from build123d import *

# Parameters (mm, degrees)
SKETCH1_W      = 11.90625
SKETCH1_H      = 34.925
EXTRUDE1_DEPTH = 1.984375
SKETCH4_W      = 11.90625
SKETCH4_H      = 11.303912273
EXTRUDE3_DEPTH = 0.79375
SKETCH2_R      = 2.1
EXTRUDE2_DEPTH = 1.984375
CHAMFER1_SIZE  = 0.508


with BuildPart() as part:
    # Sketch1 → Extrude1 (new body)
    with BuildSketch(Plane(origin=(0, 0, 0), x_dir=(1, 0, 0), z_dir=(0, 1, 0))):
        Rectangle(SKETCH1_W, SKETCH1_H)
    extrude(amount=EXTRUDE1_DEPTH)

    # Sketch4 → Extrude3 (cut)
    with BuildSketch(Plane.XZ):
        with Locations((0, 11.810543864)):
            Rectangle(SKETCH4_W, SKETCH4_H)
    extrude3 = extrude(amount=-EXTRUDE3_DEPTH, mode=Mode.SUBTRACT)

    # Mirror1: Extrude3 across plane
    add(extrude3.mirror(Plane.XY), mode=Mode.SUBTRACT)

    # Sketch2 → Extrude2 (cut)
    with BuildSketch(Plane(origin=(0, 1.984375, 0), x_dir=(1, 0, 0), z_dir=(0, 1, 0))):
        with Locations(Location((0, 12.7, 0), (0, 0, 270))):
            Circle(SKETCH2_R)
        with Locations(Location((0, -12.7, 0), (0, 0, 270))):
            Circle(SKETCH2_R)
    extrude(amount=-EXTRUDE2_DEPTH, mode=Mode.SUBTRACT)

    # Chamfer1
    chamfer1_edges = [part.edges().sort_by_distance(p)[0] for p in [
        (0, 0.79375, -14.8),
        (0, 0.79375, 10.6),
    ]]
    chamfer(chamfer1_edges, length=CHAMFER1_SIZE)


solid = part.part
CAD build for the part. Positions are in the model's coordinates, mm. A direction names the side the tool comes from. Give positions to 0.01 mm unless a question says otherwise; leave off trailing zeros. Write each loop counter-clockwise with the first axis right and the second up, starting at its lowest first coordinate (ties: lowest second). Pieces come first, ordered by that corner, then holes. Notation, with made-up numbers: M 54,84.5 L 77,84.5 A31 cw 77,118.5 Z; hole C -6.5,89 d9. An arc over 180 degrees is marked long. Put each result on its own line as item: value. Start each with the question number.
(1) Band-saw the part on D-D, the plane x = -4.5. Write the cut outline in (y, z), and give its area (3 significant figures).
(2) Mould opens along Z. For faces 1 (the face through (0.631, 1.648, -10.697)), 2 (the face through (0, 1.984, 0)), 3 (the face through (0.631, 1.648, 14.703)), 4 (the face through (0, 1, -17.462)) say: +Z half, -Z half, draft (parallel to the pull), parting line (faces both ways), or undercut.
(3) Band-saw the part on A-A, the plane z = -12.7. Write the cut outline in (x, y).
(4) Band-saw the part on B-B, the plane x = 0. Write the cut outline in (y, z), and give its area (3 significant figures).
(5) Which spindle directions (+Z, -Z, +X, -X, +Y, -Y) get a long thin tool onto all of the face, cutting with end or side? Do faces 5 (the face through (0, 0.794, -9)), 6 (the face through (0, 0, 0)), 7 (the face through (0, 0.794, 9)). Say none if no direction does.
(6) Probe L1, parallel to Z at x = 1.25, y = 1.65; L2, parallel to Z at x = 1, y = 1.6; L3, parallel to X at y = 1.6, z = 12.7. List the from-to ranges inside material, lowest first.
(7) Flat gauge pin, fed straight in: pin 1 Ø4 at (x, z) = (0, 12.7) entering from -Y. Where does the tip first touch, or does it go through?
(8) Band-saw the part on C-C, the plane y = 1.65. Write the cut outline in (x, z), and give its area (3 significant figures).
Response values:
1. outline: M 0,-6.16 L 0.79,-6.16 L 0.79,-17.46 L 1.98,-17.46 L 1.98,17.46 L 0.79,17.46 L 0.79,6.16 L 0,6.16 Z
1. area: 51.4 mm2
2. face 1: undercut
2. face 2: draft
2. face 3: undercut
2. face 4: -Z half
3. outline: M -5.95,0.79 L -2.61,0.79 L -2.1,1.3 L -2.1,1.98 L -5.95,1.98 Z; M 2.1,1.3 L 2.61,0.79 L 5.95,0.79 L 5.95,1.98 L 2.1,1.98 Z
4. outline: M 0,-6.16 L 0.79,-6.16 L 0.79,-10.09 L 1.3,-10.6 L 1.98,-10.6 L 1.98,10.6 L 1.3,10.6 L 0.79,10.09 L 0.79,6.16 L 0,6.16 Z; M 0.79,-17.46 L 1.98,-17.46 L 1.98,-14.8 L 1.3,-14.8 L 0.79,-15.31 Z; M 0.79,15.31 L 1.3,14.8 L 1.98,14.8 L 1.98,17.46 L 0.79,17.46 Z
4. area: 40.8 mm2
5. face 5: -Z, +X, -X, -Y
5. face 6: +Z, -Z, +X, -X, -Y
5. face 7: +Z, +X, -X, -Y
6. L1: z = -17.46 to -14.39, -11.01 to 11.01, 14.39 to 17.46
6. L2: z = -17.46 to -14.55, -10.85 to 10.85, 14.55 to 17.46
6. L3: x = -5.95 to -2.1, 2.1 to 5.95
7. pin 1: passes through
8. outline: M -5.95,-17.46 L 5.95,-17.46 L 5.95,17.46 L -5.95,17.46 Z; hole C 0,-12.7 d4.2; hole C 0,12.7 d4.2
8. area: 388 mm2
